Source: CAD feature listing. Evaluate the final solid. Frame: model axes, mm. A direction names the side the tool comes from. Coordinates: 2 decimals unless noted, no trailing zeros. Loops run counter-clockwise (first coordinate to the right, second up) from the corner with the lowest first, then second, coordinate; pieces in that order, holes last. Notation, with made-up numbers: (26, 83.25) -> (48, 83.25) arc R7 cw to (48, 92.25) -> close; hole circle Ø6 at (-38, 49.25). An arc over 180 degrees is marked (long way). Answer as a JSON object with one key per item and string values. Group by question number.
from build123d import *

# Parameters (mm, degrees)
SKETCH_1_R          = 12.2
EXTRUDE_4_DEPTH     = 36.5
SKETCH_10_R         = 1
EXTRUDE_7_DEPTH     = 11
SKETCH_11_R         = 3.225
EXTRUDE_8_DEPTH     = 0.5
SKETCH_13_R         = 1.5
CUT_EXTRUDE_2_DEPTH = 3


with BuildPart() as part:
    # 草图1 → 凸台-拉伸4 (new body)
    with BuildSketch(Plane.XY):
        Circle(SKETCH_1_R)
    extrude(amount=EXTRUDE_4_DEPTH)

    # 草图10 → 凸台-拉伸7 (add)
    with BuildSketch(Plane(origin=(0, 0, 0), x_dir=(-1, 0, 0), z_dir=(0, 0, -1))):
        with Locations(Location((0, 0, 0), (0, 0, 180))):
            Circle(SKETCH_10_R)
    extrude(amount=EXTRUDE_7_DEPTH)

    # 草图11 → 凸台-拉伸8 (add)
    with BuildSketch(Plane(origin=(0, 0, 0), x_dir=(-1, 0, 0), z_dir=(0, 0, -1))):
        with Locations(Location((0, 0, 0), (0, 0, 180))):
            Circle(SKETCH_11_R)
    extrude(amount=EXTRUDE_8_DEPTH)

    # 草图13 → 切除-拉伸2 (cut)
    with BuildSketch(Plane(origin=(0, 0, 0), x_dir=(-1, 0, 0), z_dir=(0, 0, -1))):
        with Locations((0, 8.504557186)):
            Circle(SKETCH_13_R)
        with Locations((0, -8.512012438)):
            Circle(SKETCH_13_R)
    extrude(amount=-CUT_EXTRUDE_2_DEPTH, mode=Mode.SUBTRACT)


solid = part.part
1. Section query D-D on x = -2.75. Return loops of the section in (y, z), then the cut area to 3 significant figures.
2. Section query B-B on x = 0. Return loops of the section in (y, z) (3 decimals), then the cut area to 3 significant figures.
3. Pin query (flat end, axial travel): pin 1 Ø2 at (y, z) = (-7, 13) entering from +X; pin 2 Ø1 at (x, y) = (8, -5) entering from -Z; pin 3 Ø2.5 at (x, y) = (0, 8.5) entering from -Z; pin 4 Ø10 at (x, z) = (-5, 28.5) entering from +Y. Return the tip coordinate at first contact, or that it passes through.
4. Mould query, pull axis Y, two halves, no side actions, for faces 3 (the face through (0, 0, -11)), 4 (the face through (0, 1, -6)), 5 (the face through (0, 9, 3)). Classes: pulls with the +Y half, pulls with the -Y half, needs draft (parallel to the pull), parting line crosses it, or undercut.
5. Reachability of faces 1 (the face through (-12.19, 0.54, 17.99)), 2 (the face through (0.325, -9.976, 1.479)) from +Z, -Z, +X, -X, +Y, -Y: full face, straight path, thin tool, end or side. Return the list, or none.
6. Section query A-A on y = 0. Return loops of the section in (x, z) (3 decimals).
7. Ray query, L1, parallel to Y at x = 0, z = 1.2; L2, parallel to Z at x = 7.5, y = -9.5; L3, parallel to Y at x = -0.25, z = 20. Return the intervals inside material, ascending.
8. Section query C-C on z = 17. Return loops of the section in (x, y).
Solved:
{
 "1": {"outline": "(-11.89, 0) -> (-1.68, 0) -> (-1.68, -0.5) -> (1.68, -0.5) -> (1.68, 0) -> (11.89, 0) -> (11.89, 36.5) -> (-11.89, 36.5) -> close", "area": "869 mm^2"},
 "2": {"outline": "(-12.2, 0) -> (-10.012, 0) -> (-10.012, 3) -> (-7.012, 3) -> (-7.012, 0) -> (-3.225, 0) -> (-3.225, -0.5) -> (-1, -0.5) -> (-1, -11) -> (1, -11) -> (1, -0.5) -> (3.225, -0.5) -> (3.225, 0) -> (7.005, 0) -> (7.005, 3) -> (10.005, 3) -> (10.005, 0) -> (12.2, 0) -> (12.2, 36.5) -> (-12.2, 36.5) -> close", "area": "897 mm^2"},
 "3": {"pin 1": "x = 10.62", "pin 2": "z = 0", "pin 3": "z = 3", "pin 4": "y = 12.2"},
 "4": {"face 3": "needs draft", "face 4": "parting line crosses it", "face 5": "undercut"},
 "5": {"face 1": "+Z, -Z", "face 2": "-Z"},
 "6": {"outline": "(-12.2, 0) -> (-3.225, 0) -> (-3.225, -0.5) -> (-1, -0.5) -> (-1, -11) -> (1, -11) -> (1, -0.5) -> (3.225, -0.5) -> (3.225, 0) -> (12.2, 0) -> (12.2, 36.5) -> (-12.2, 36.5) -> close"},
 "7": {"L1": "-12.2 to -10.01, -7.01 to 7, 10 to 12.2", "L2": "0 to 36.5", "L3": "-12.2 to 12.2"},
 "8": {"outline": "circle Ø24.4 at (0, 0)"}
}
